```python
from build123d import *

# Parameters (mm, degrees)
F1_DEPTH    = 250
F2_W        = 38
F2_H        = 13
F3_DEPTH    = 250
F4_T1_DEPTH = 509.3674969976
F5_R        = 9
F6_R        = 1
F8_DEPTH    = 250


# Not quite as in the source:
# - a fillet or chamfer that OpenCascade refuses, or shapes differently, is made with other operations: its cross-section is extruded or revolved along the edge and cut away or added


with BuildPart() as f1:
    # F0 (on Front) → F1 (new body, symmetric)
    with BuildSketch(Plane.XZ):
        with BuildLine():
            Line((22.5, 0), (0, 0))
            Line((0, 0), (-22.5, 0))
            Line((-22.5, 0), (-22.5, 1.3))
            Line((-22.5, 1.3), (-45.5824640741, 1.3))
            Line((-45.5824640741, 1.3), (-57.5, -8.7))
            Line((-57.5, -8.7), (-57.5, -12.7))
            Line((-57.5, -12.7), (-40.1794919243, -22.7))
            ThreePointArc((-40.1794919243, -22.7), (0, -18.6224551416), (40.1794919243, -22.7))
            Line((40.1794919243, -22.7), (57.5, -12.7))
            Line((57.5, -12.7), (57.5, -8.7))
            Line((57.5, -8.7), (45.5824640741, 1.3))
            Line((45.5824640741, 1.3), (22.5, 1.3))
            Line((22.5, 1.3), (22.5, 0))
        make_face()
    extrude(amount=F1_DEPTH, both=True)

    # F2 (on Front) → F3 (cut, symmetric)
    with BuildSketch(Plane.XZ):
        with Locations((0, -8.5)):
            Rectangle(F2_W, F2_H)
    extrude(amount=F3_DEPTH, both=True, mode=Mode.SUBTRACT)

    # F4: fillet of radius 2 on 2 edges, made by hand

    # F4_s2 → F4_t1 (cut)
    with BuildSketch(Plane.XZ.offset(-254.6837484988)):
        with BuildLine():
            ThreePointArc((24.3734993995, 1.3), (23.2333239744, 0.9431676725), (22.5, 0))
            Line((22.5, 0), (22.5, 1.3))
            Line((22.5, 1.3), (24.3734993995, 1.3))
        make_face()
        with BuildLine():
            ThreePointArc((-24.3734993995, 1.3), (-23.2333239744, 0.9431676725), (-22.5, 0))
            Line((-22.5, 0), (-22.5, 1.3))
            Line((-22.5, 1.3), (-24.3734993995, 1.3))
        make_face()
    extrude(amount=F4_T1_DEPTH, mode=Mode.SUBTRACT)

    # F5
    f5_edges = [f1.edges().sort_by_distance(p)[0] for p in [
        (45.582464, 0, 1.3),
        (-45.582464, 0, 1.3),
        (40.179492, 0, -22.7),
        (-40.179492, 0, -22.7),
    ]]
    fillet(f5_edges, radius=F5_R)

    # F6
    f6_edges = [f1.edges().sort_by_distance(p)[0] for p in [
        (57.5, 0, -8.7),
        (57.5, 0, -12.7),
        (-57.5, 0, -8.7),
        (-57.5, 0, -12.7),
    ]]
    fillet(f6_edges, radius=F6_R)

    # F7 (on Front) → F8 (cut, symmetric)
    with BuildSketch(Plane.XZ):
        with BuildLine():
            ThreePointArc((-42.1022690923, -19.2804830077), (-39.7790673433, -20.1186780608), (-37.3093701274, -20.0978700124))
            ThreePointArc((-37.3093701274, -20.0978700124), (-29.1789785809, -18.7410222645), (-21, -17.7170047426))
            Line((-21, -17.7170047426), (-21, -2))
            Line((-21, -2), (-22.5, -2))
            ThreePointArc((-22.5, -2), (-23.2333239744, -1.0568323275), (-24.3734993995, -0.7))
            Line((-24.3734993995, -0.7), (-42.3067319657, -0.7))
            ThreePointArc((-42.3067319657, -0.7), (-44.7008729689, -1.1221516545), (-46.8062452335, -2.3376888982))
            Line((-46.8062452335, -2.3376888982), (-54.6622869129, -8.9296905739))
            ThreePointArc((-54.6622869129, -8.9296905739), (-55.3691010897, -10.6360909457), (-54.3767116936, -12.1938302677))
            Line((-54.3767116936, -12.1938302677), (-42.1022690923, -19.2804830077))
        make_face()
        with BuildLine():
            Line((42.3067319657, -0.7), (24.3734993995, -0.7))
            ThreePointArc((24.3734993995, -0.7), (23.2333239744, -1.0568323275), (22.5, -2))
            Line((22.5, -2), (21, -2))
            Line((21, -2), (21, -17.7170047426))
            ThreePointArc((21, -17.7170047426), (29.1789785809, -18.7410222645), (37.3093701274, -20.0978700124))
            ThreePointArc((37.3093701274, -20.0978700124), (39.7790673433, -20.1186780608), (42.1022690923, -19.2804830077))
            Line((42.1022690923, -19.2804830077), (54.3767116936, -12.1938302677))
            ThreePointArc((54.3767116936, -12.1938302677), (55.3691010897, -10.6360909457), (54.6622869129, -8.9296905739))
            Line((54.6622869129, -8.9296905739), (46.8062452335, -2.3376888982))
            ThreePointArc((46.8062452335, -2.3376888982), (44.7008729689, -1.1221516545), (42.3067319657, -0.7))
        make_face()
    extrude(amount=F8_DEPTH, both=True, mode=Mode.SUBTRACT)


solid = f1.part
```
Geometry check sheet. Reference: the model listing, model coordinates, mm. A direction names the side the tool comes from. Round coordinates to 2 decimals unless told otherwise and drop trailing zeros. Loops run counter-clockwise (first coordinate to the right, second up) from the corner with the lowest first, then second, coordinate; pieces in that order, holes last. Notation, with made-up numbers: (66.5, 12.5) - (88.5, 12.5) arc R32 cw to (88.5, 38.5) - close; hole circle Ø9 at (-21.5, 64). An arc over 180 degrees is marked (long way). Use a Markdown table: item, result.
Q1. Access from +Z, -Z, +X, -X, +Y, -Y to the whole of each face (thin tool, end or side, straight path). Record for faces 1 (the cylindrical face through (-0.52, -3.5, -18.623)), 2 (the flat face through (-50.68, 3.5, -5.59)), 3 (the flat face through (0, -4, 0)).
Solutions:
| item | result |
|---|---|
| face 1 | -Z, +Y, -Y |
| face 2 | +Y, -Y |
| face 3 | +Z, +Y, -Y |
Q2. Cross-section at B-B on y = 66. State how many separate pieces and enclosed holes the cut face has, plus the area to 3 significant figures.
Solutions:
| item | result |
|---|---|
| separate pieces | 1 |
| enclosed holes | 3 |
| area | 623 mm2 |
Q3. Go/stop test with flat-tipped pins: P1, Ø11.5, axis at x = 8.5, y = -104.5, coming from the -Z side; P2, Ø12, axis at x = 23.5, y = -85, coming from the -Z side; P3, Ø3, axis at x = -12.5, y = 146, coming from the +Z side. Record where each tip stops, or that it passes through.
Solutions:
| item | result |
|---|---|
| P1 | stops at z = -19.13 |
| P2 | stops at z = -20.81 |
| P3 | stops at z = 0 |
Q4. Cross-section at C-C on x = -10. Record the cut outline in (y, z), plus the area to 3 significant figures.
Solutions:
| item | result |
|---|---|
| outline | (-250, -18.87) - (250, -18.87) - (250, -15) - (-250, -15) - close; (-250, -2) - (250, -2) - (250, 0) - (-250, 0) - close |
| area | 2,940 mm2 |
Q5. Material ranges on line 1 (X direction, y = -28, z = -9); line 2 (Z direction, x = 15.5, y = 51); line 3 (X direction, y = 14.5, z = -6.75), recorded low to high.
Solutions:
| item | result |
|---|---|
| line 1 | x = -57.49 to -54.74, -21 to -19, 19 to 21, 54.74 to 57.49 |
| line 2 | z = -19.22 to -15, -2 to 0 |
| line 3 | x = -55.18 to -52.06, -21 to -19, 19 to 21, 52.06 to 55.18 |
Q6. Draft check along X on faces 4 (the flat face through (48.15, -3.5, -15.79)), 5 (the flat face through (-50.148, -3.5, -16.944)), 6 (the flat face through (52.681, -3.5, -4.656)). Enter one of: released by +X, released by -X, zero draft, split by the parting line, or undercut.
Solutions:
| item | result |
|---|---|
| face 4 | undercut |
| face 5 | released by -X |
| face 6 | released by +X |
Q7. Cross-section at A-A on x = 12.5. Record the cut outline in (y, z).
Solutions:
| item | result |
|---|---|
| outline | (-250, -19.01) - (250, -19.01) - (250, -15) - (-250, -15) - close; (-250, -2) - (250, -2) - (250, 0) - (-250, 0) - close |
